```python
from build123d import *

# Parameters (mm, degrees)
F0_W     = 152.4
F0_H     = 25.4
F1_DEPTH = 1.5875
F3_DEPTH = 1.5885
F4_W     = 71.12
F4_H     = 25.4
F5_DEPTH = 1.5885
F6_W     = 2.54
F6_H     = 5.08
F7_DEPTH = 1.5875


with BuildPart() as f1:
    # F0 (on Front) → F1 (new body)
    with BuildSketch(Plane.XZ):
        with Locations((76.2, 12.7)):
            Rectangle(F0_W, F0_H)
    extrude(amount=F1_DEPTH)

    # F2 (on Front) → F3 (cut, through all)
    with BuildSketch(Plane.XZ):
        Polygon((4.2926, 5.08), (2.54, 0), (7.62, 0), (5.8674, 5.08), (5.8674, 12.7), (4.2926, 12.7), align=None)
        Polygon((14.4526, 5.08), (12.7, 0), (17.78, 0), (16.0274, 5.08), (16.0274, 12.7), (14.4526, 12.7), align=None)
        Polygon((24.6126, 5.08), (22.86, 0), (27.94, 0), (26.1874, 5.08), (26.1874, 12.7), (24.6126, 12.7), align=None)
        Polygon((34.7726, 5.08), (33.02, 0), (38.1, 0), (36.3474, 5.08), (36.3474, 12.7), (34.7726, 12.7), align=None)
        Polygon((44.9326, 5.08), (43.18, 0), (48.26, 0), (46.5074, 5.08), (46.5074, 12.7), (44.9326, 12.7), align=None)
        Polygon((55.0926, 5.08), (53.34, 0), (58.42, 0), (56.6674, 5.08), (56.6674, 12.7), (55.0926, 12.7), align=None)
        Polygon((65.2526, 5.08), (63.5, 0), (68.58, 0), (66.8274, 5.08), (66.8274, 12.7), (65.2526, 12.7), align=None)
        Polygon((75.4126, 5.08), (73.66, 0), (78.74, 0), (76.9874, 5.08), (76.9874, 12.7), (75.4126, 12.7), align=None)
    extrude(amount=F3_DEPTH, mode=Mode.SUBTRACT)

    # F4 (on face) → F5 (cut, through all)
    with BuildSketch(Plane.XZ.offset(1.5875)):
        with Locations((116.84, 12.7)):
            Rectangle(F4_W, F4_H)
    extrude(amount=-F5_DEPTH, mode=Mode.SUBTRACT)

    # F6 (on face) → F7 (join, through all)
    with BuildSketch(Plane.XZ.offset(1.5875)):
        with Locations((1.27, -2.54)):
            Rectangle(F6_W, F6_H)
        with Locations((80.01, -2.54)):
            Rectangle(F6_W, F6_H)
    extrude(amount=-F7_DEPTH)


solid = f1.part
```
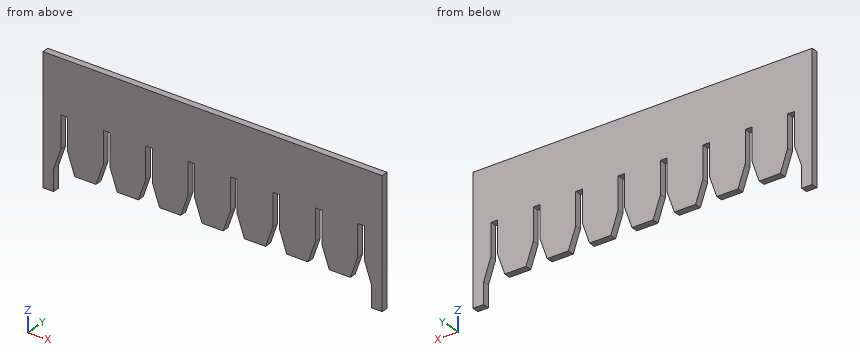
Could you check a few things on this model? Use its own coordinates, in mm. Coordinates: 2 decimals unless noted, no trailing zeros. Write each loop counter-clockwise with the first axis right and the second up, starting at its lowest first coordinate (ties: lowest second). Pieces come first, ordered by that corner, then holes. Notation, with made-up numbers: (-15.5, 20) -> (12.5, 20) arc R35 ccw to (12.5, 57) -> close; hole circle Ø4 at (37, 85.25). An arc over 180 degrees is marked (long way). Write item = value, one per line. Start each with the question number.
(1) I want a section at A-A (z = -1). Please give me the cut outline in (x, y).
(2) I need wall thicknesses on line 1 (X direction, y = -1.1, z = -1.5); line 2 (Z direction, x = 10.5, y = -0.4); line 3 (Z direction, x = 55.5, y = -0.6). Which ranges of each line are inside material? Lowest first, please. Write a range as [from, to].
(3) I want a section at C-C (x = 9). Please give me the cut outline in (y, z).
(4) Will this pin go through, and if not, where does the flat tip stop? pin 1 (0.5 mm diameter, centred on x = 15.5, y = -1, fed in from -Z).
(5) I want a section at B-B (z = 7). Give the number of separate pieces and of enclosed holes in the cut face, plus the area to 3 significant figures.
Result set:
q1.outline = (0, -1.59) -> (2.54, -1.59) -> (2.54, 0) -> (0, 0) -> close; (78.74, -1.59) -> (81.28, -1.59) -> (81.28, 0) -> (78.74, 0) -> close
q2.line_1 = [0, 2.54], [78.74, 81.28]
q2.line_2 = [0, 25.4]
q2.line_3 = [12.7, 25.4]
q3.outline = (-1.59, 0) -> (0, 0) -> (0, 25.4) -> (-1.59, 25.4) -> close
q4.pin_1 = 12.7
q5.separate_pieces = 9
q5.enclosed_holes = 0
q5.area = 109 mm2
